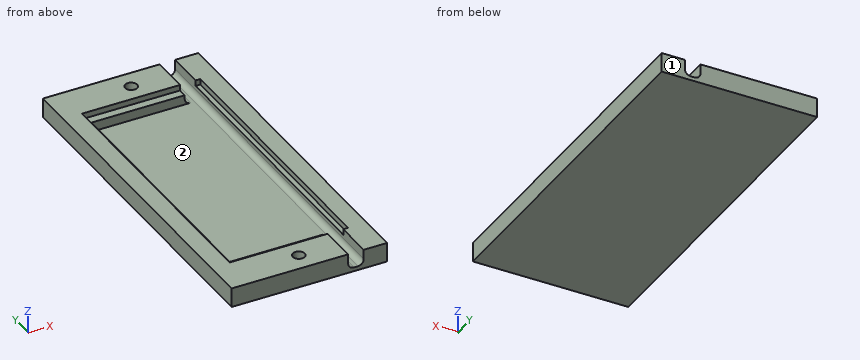
```python
from build123d import *

# Parameters (mm, degrees)
SKETCH1_W           = 90
SKETCH1_H           = 40
BOSS_EXTRUDE1_DEPTH = 5
SKETCH2_W           = 30.5
SKETCH2_H           = 70.5
CUT_EXTRUDE1_DEPTH  = 1.5
SKETCH3_W           = 28
SKETCH3_H           = 66
CUT_EXTRUDE2_DEPTH  = 2.5
SKETCH4_W           = 4
SKETCH4_H           = 4
CUT_EXTRUDE3_DEPTH  = 99.615414617
FILLET1_R           = 1.5
SKETCH6_R           = 1.55
CUT_EXTRUDE5_DEPTH  = 4.5
SKETCH7_R           = 1.55
CUT_EXTRUDE6_DEPTH  = 4.5


with BuildPart() as part:
    # Sketch1 → Boss-Extrude1 (new body)
    with BuildSketch(Plane(origin=(0, 0, 0), x_dir=(0, 1, 0), z_dir=(0, 0, 1))):
        with Locations((45, 20)):
            Rectangle(SKETCH1_W, SKETCH1_H)
    extrude(amount=BOSS_EXTRUDE1_DEPTH)

    # Sketch2 → Cut-Extrude1 (cut)
    with BuildSketch(Plane.XY.offset(5)):
        with Locations((-20, 45)):
            Rectangle(SKETCH2_W, SKETCH2_H)
    extrude(amount=-CUT_EXTRUDE1_DEPTH, mode=Mode.SUBTRACT)

    # Sketch3 → Cut-Extrude2 (cut)
    with BuildSketch(Plane.XY.offset(3.5)):
        with Locations((-20, 45)):
            Rectangle(SKETCH3_W, SKETCH3_H)
    extrude(amount=-CUT_EXTRUDE2_DEPTH, mode=Mode.SUBTRACT)

    # Sketch4 → Cut-Extrude3 (cut, through all)
    with BuildSketch(Plane.XZ):
        with Locations((-8, 3)):
            Rectangle(SKETCH4_W, SKETCH4_H)
    extrude(amount=-CUT_EXTRUDE3_DEPTH, mode=Mode.SUBTRACT)

    # Fillet1
    fillet1_edges = [part.edges().sort_by_distance(p)[0] for p in [
        (-6, 45, 1),
        (-10, 84, 1),
        (-10, 6, 1),
    ]]
    fillet(fillet1_edges, radius=FILLET1_R)

    # Sketch6 → Cut-Extrude5 (cut)
    with BuildSketch(Plane.XY.offset(5)):
        with Locations((-20, 85)):
            Circle(SKETCH6_R)
    extrude(amount=-CUT_EXTRUDE5_DEPTH, mode=Mode.SUBTRACT)

    # Sketch7 → Cut-Extrude6 (cut)
    with BuildSketch(Plane.XY.offset(5)):
        with Locations((-20, 5)):
            Circle(SKETCH7_R)
    extrude(amount=-CUT_EXTRUDE6_DEPTH, mode=Mode.SUBTRACT)


solid = part.part
```
Could you check a few things on this model? Use its own coordinates, in mm. Face numbers are marked on the shaded views. Coordinates: 2 decimals unless noted, no trailing zeros. Write each loop counter-clockwise with the first axis right and the second up, starting at its lowest first coordinate (ties: lowest second). Pieces come first, ordered by that corner, then holes. Notation, with made-up numbers: (82, -21) -> (110, -21) arc R24 cw to (110, -7) -> close; hole circle Ø3 at (73.5, 44.5). An arc over 180 degrees is marked (long way). One line per question, with ' | ' between items. Start each with the question number.
1. If we section it at B-B (y = 74): Please give me the cut outline in (x, z).
2. Thinking about a two-plate mould opening in X: for the marked faces 1 and 2, which applies, pulls with the +X half, pulls with the -X half, needs draft (parallel to the pull), parting line crosses it, or undercut?
3. Please list where these lines run through material, in increasing order: line 1 along Y through (x, z) = (-20, 1.7); line 2 along X through (y, z) = (85, 2.95); line 3 along Y through (x, z) = (-20, 3.95).
4. If we section it at A-A (x = -12): Please give me the cut outline in (y, z).
5. If we section it at C-C (z = 1.75): Please give me the cut outline in (x, y), and give its area (3 significant figures).
6. If we section it at D-D (x = -20): Please give me the cut outline in (y, z).
7. Will these pins go through, and if not, where does the flat tip stop? P1, Ø7.5, axis at x = -21.5, y = 59.5, coming from the +Z side; P2, Ø1.5, axis at x = -20, y = 85.5, coming from the +Z side.
Return value:
1) outline: (-40, 0) -> (0, 0) -> (0, 5) -> (-4.75, 5) -> (-4.75, 3.5) -> (-6, 3.5) -> (-6, 2.5) arc R1.5 cw to (-7.5, 1) -> (-34, 1) -> (-34, 3.5) -> (-35.25, 3.5) -> (-35.25, 5) -> (-40, 5) -> close
2) face 1: needs draft | face 2: undercut
3) line 1: y = 0 to 3.45, 6.55 to 12, 78 to 83.45, 86.55 to 90 | line 2: x = -40 to -21.55, -18.45 to -10, -6 to 0 | line 3: y = 0 to 3.45, 6.55 to 9.75, 80.25 to 83.45, 86.55 to 90
4) outline: (0, 0) -> (90, 0) -> (90, 5) -> (80.25, 5) -> (80.25, 3.5) -> (78, 3.5) -> (78, 1) -> (12, 1) -> (12, 3.5) -> (9.75, 3.5) -> (9.75, 5) -> (0, 5) -> close
5) outline: (-40, 0) -> (-9.8, 0) -> (-9.8, 12) -> (-34, 12) -> (-34, 78) -> (-9.8, 78) -> (-9.8, 90) -> (-40, 90) -> close; (-6.2, 0) -> (0, 0) -> (0, 90) -> (-6.2, 90) -> close; hole circle Ø3.1 at (-20, 5); hole circle Ø3.1 at (-20, 85) | area: 1,660 mm²
6) outline: (0, 0) -> (90, 0) -> (90, 5) -> (86.55, 5) -> (86.55, 0.5) -> (83.45, 0.5) -> (83.45, 5) -> (80.25, 5) -> (80.25, 3.5) -> (78, 3.5) -> (78, 1) -> (12, 1) -> (12, 3.5) -> (9.75, 3.5) -> (9.75, 5) -> (6.55, 5) -> (6.55, 0.5) -> (3.45, 0.5) -> (3.45, 5) -> (0, 5) -> close
7) P1: stops at z = 1 | P2: stops at z = 0.5
